Input: part model. Units: mm. Frame: model coordinates. Face numbers are marked on the shaded views. A direction names the side the tool comes from. Coordinates: 2 decimals unless noted, no trailing zeros. Order: outer loops, then holes, each group sorted by start corner. A loop starts at its lowest first (then second) coordinate and runs counter-clockwise, first axis right, second up. Notation, with made-up numbers: M -4,26.5 L 12,26.5 A23 ccw 12,50.5 Z; hole C 77,62 d1. An arc over 180 degrees is marked long. One line per item, written item: value.
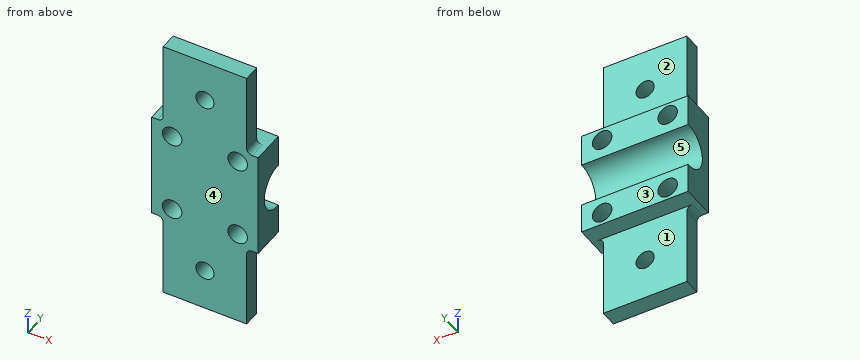
```python
from build123d import *

# Parameters (mm, degrees)
SKETCH1_W                            = 38.29
SKETCH1_H                            = 38.3
BOSS_EXTRUDE1_DEPTH                  = 12.12
SKETCH2_R                            = 8
CUT_EXTRUDE1_DEPTH                   = 45.494280531
M8X1_0_TAPPED_HOLE2_D                = 7
MIRROR1_AT_THE_SECOND_PLANE_COPY_1_D = 7
SKETCH9_W                            = 30
SKETCH9_H                            = 30
SKETCH9_R                            = 3.25
BOSS_EXTRUDE2_DEPTH                  = 6
FILLET1_R                            = 2


with BuildPart() as part:
    # Sketch1 → Boss-Extrude1 (new body)
    with BuildSketch(Plane(origin=(0, 0, 0), x_dir=(1, 0, 0), z_dir=(0, 1, 0))):
        Rectangle(SKETCH1_W, SKETCH1_H)
    extrude(amount=BOSS_EXTRUDE1_DEPTH)

    # Sketch2 → Cut-Extrude1 (cut, through all)
    with BuildSketch(Plane(origin=(19.145, 0, 0), x_dir=(0, 0, -1), z_dir=(1, 0, 0))):
        with Locations((0.363834185, 11.62)):
            Circle(SKETCH2_R)
    extrude(amount=-CUT_EXTRUDE1_DEPTH, mode=Mode.SUBTRACT)

    # M8x1.0 Tapped Hole2 (through all)
    with Locations(Plane(origin=(0, 12.12, 0), x_dir=(1, 0, 0), z_dir=(0, 1, 0))):
        with Locations((-11.77, 14.55), (11.77, 14.55), (-11.77, -14.55), (11.77, -14.55)):
            m8x1_0_tapped_hole2 = Hole(M8X1_0_TAPPED_HOLE2_D / 2)

    # Mirror1: M8x1.0 Tapped Hole2 across plane
    add(m8x1_0_tapped_hole2.mirror(Plane.XY), mode=Mode.SUBTRACT)

    # Mirror1 at the second plane: M8x1.0 Tapped Hole2 across plane
    add(m8x1_0_tapped_hole2.mirror(Plane(origin=(0, 0, 0), x_dir=(0, 0, 1), z_dir=(1, 0, 0))), mode=Mode.SUBTRACT)

    # Mirror1 at the second plane copy 1 (through all)
    with Locations(Plane(origin=(0, 12.12, 0), x_dir=(-1, 0, 0), z_dir=(0, 1, 0))):
        with Locations((-11.77, 14.55), (11.77, 14.55), (-11.77, -14.55), (11.77, -14.55)):
            Hole(MIRROR1_AT_THE_SECOND_PLANE_COPY_1_D / 2)

    # Sketch9 → Boss-Extrude2 (add)
    with BuildSketch(Plane.XZ):
        with Locations((0, -34.15)):
            Rectangle(SKETCH9_W, SKETCH9_H)
        with Locations(Location((0, -34.15, 0), (0, 0, 270))):
            Circle(SKETCH9_R, mode=Mode.SUBTRACT)
    boss_extrude2 = extrude(amount=-BOSS_EXTRUDE2_DEPTH)

    # Mirror2: Boss-Extrude2 across plane
    add(boss_extrude2.mirror(Plane.XY))

    # Fillet1
    fillet1_edges = [part.edges().sort_by_distance(p)[0] for p in [
        (15, 3, 19.15),
        (-15, 3, 19.15),
        (15, 3, -19.15),
        (-15, 3, -19.15),
    ]]
    fillet(fillet1_edges, radius=FILLET1_R)


solid = part.part
```
(1) Ray query, line 1 (X direction, y = 6, z = -14.55) (3 decimals); line 2 (Z direction, x = -12, y = 2.5); line 3 (X direction, y = 3.45, z = -34.15). Return the intervals inside material, ascending. Write a range as from..to.
Data:
line 1: x = -19.145..-15.27, -8.27..8.27, 15.27..19.145
line 2: z = -49.15..-18.04, -11.06..11.06, 18.04..49.15
line 3: x = -15..-3.25, 3.25..15
(2) Cut plane D-D on y = 2.5. Output: boundary loops of the cut face in (x, z) (3 decimals).
Data:
outline: M -19.145,-19.15 L -17,-19.15 A2 cw -15,-21.15 L -15,-49.15 L 15,-49.15 L 15,-21.15 A2 cw 17,-19.15 L 19.145,-19.15 L 19.145,19.15 L 17,19.15 A2 cw 15,21.15 L 15,49.15 L -15,49.15 L -15,21.15 A2 cw -17,19.15 L -19.145,19.15 Z; hole C -11.77,-14.55 d7; hole C -11.77,14.55 d7; hole C 0,-34.15 d6.5; hole C 0,34.15 d6.5; hole C 11.77,-14.55 d7; hole C 11.77,14.55 d7
(3) Draft query along Z for the marked faces 4 and 5. Return one class per face: released by +Z, released by -Z, zero draft, split by the parting line, or undercut.
Data:
face 4: zero draft
face 5: undercut
(4) Cut plane A-A on z = -14.55. Output: boundary loops of the cut face in (x, y) (3 decimals).
Data:
outline: M -19.145,0 L -15.27,0 L -15.27,12.12 L -19.145,12.12 Z; M -8.27,0 L 8.27,0 L 8.27,12.12 L -8.27,12.12 Z; M 15.27,0 L 19.145,0 L 19.145,12.12 L 15.27,12.12 Z
(5) Access query for the marked faces 1, 2 and 3. Directions: +Z, -Z, +X, -X, +Y, -Y. A direction counts if a zero-diameter tool reaches every point of the face in a straight line with its end or side. Return the directions, or none.
Data:
face 1: -Z, +X, -X, +Y
face 2: +Z, +X, -X, +Y
face 3: +Z, -Z, +X, -X, +Y
(6) First-contact query: pin 1 (5 mm diameter, centred on y = 3.5, z = 38.5, fed in from -X); pin 2 (7.5 mm diameter, centred on x = 0, z = 34.15, fed in from +Y); pin 3 (1.8 mm diameter, centred on y = 3.5, z = -29.5, fed in from +X). Flat tips, straight axial feed; report the tip coordinate or a pass-through.
Data:
pin 1: stops at x = -15
pin 2: stops at y = 6
pin 3: stops at x = 15
(7) Cut plane C-C on x = -11.77. Output: boundary loops of the cut face in (y, z), plus the area to 3 significant figures.
Data:
outline: M 0,-49.15 L 6,-49.15 L 6,-19.15 L 12.12,-19.15 L 12.12,-18.05 L 0,-18.05 Z; M 0,-11.05 L 12.12,-11.05 L 12.12,-8.35 A8 cw long 12.12,7.62 L 12.12,11.05 L 0,11.05 Z; M 0,18.05 L 12.12,18.05 L 12.12,19.15 L 6,19.15 L 6,49.15 L 0,49.15 Z
area: 546 mm2
(8) Cut plane B-B on y = 8.25. Output: boundary loops of the cut face in (x, z) (3 decimals).
Data:
outline: M -19.145,-19.15 L 19.145,-19.15 L 19.145,-7.619 L -19.145,-7.619 Z; M -19.145,6.892 L 19.145,6.892 L 19.145,19.15 L -19.145,19.15 Z; hole C -11.77,-14.55 d7; hole C -11.77,14.55 d7; hole C 11.77,-14.55 d7; hole C 11.77,14.55 d7
